```python
from build123d import *

# Parameters (mm, degrees)
BOSS_EXTRUDE1_DEPTH = 3
SKETCH2_W           = 30
SKETCH2_H           = 3
BOSS_EXTRUDE2_DEPTH = 24
SKETCH5_R           = 3.3
CUT_EXTRUDE1_DEPTH  = 10


with BuildPart() as part:
    # Sketch1 → Boss-Extrude1 (new body)
    with BuildSketch(Plane.XZ.offset(-12)):
        Polygon((15, 0), (15, 33), (-15, 3), (-15, 0), align=None)
    extrude(amount=-BOSS_EXTRUDE1_DEPTH)

    # Sketch2 → Boss-Extrude2 (add)
    with BuildSketch(Plane.XZ.offset(-12)):
        with Locations((0, 1.5)):
            Rectangle(SKETCH2_W, SKETCH2_H)
    extrude(amount=BOSS_EXTRUDE2_DEPTH)

    # Sketch5 → Cut-Extrude1 (cut)
    with BuildSketch(Plane(origin=(0, 0, 0), x_dir=(-1, 0, 0), z_dir=(0, 0, -1))):
        with Locations((-9, 3)):
            Circle(SKETCH5_R)
        with Locations((9, 3)):
            Circle(SKETCH5_R)
    extrude(amount=-CUT_EXTRUDE1_DEPTH, mode=Mode.SUBTRACT)


solid = part.part
```
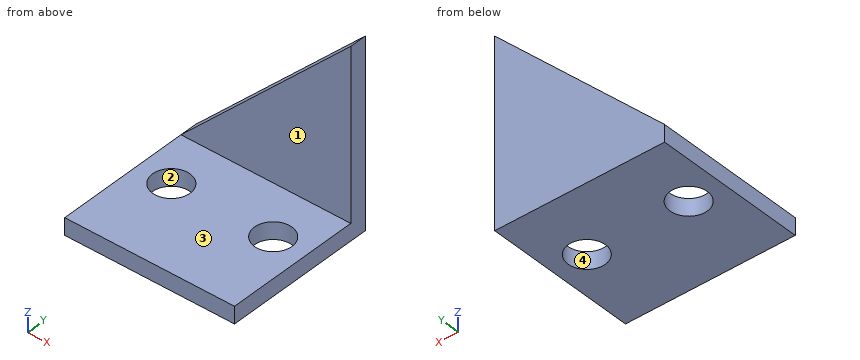
The model under review builds one solid part; all positions refer to its coordinate system, in mm. Face numbers are marked on the shaded views. A direction names the side the tool comes from. Give positions to 0.01 mm unless a question says otherwise; leave off trailing zeros. Write each loop counter-clockwise with the first axis right and the second up, starting at its lowest first coordinate (ties: lowest second). Pieces come first, ordered by that corner, then holes. Notation, with made-up numbers: (46.5, 30.25) - (84.5, 30.25) arc R24 cw to (84.5, 53.25) - close; hole circle Ø5 at (24, 80.5). An arc over 180 degrees is marked (long way). Answer in a Markdown table with one row per item. Add a question column.
1. Draft analysis for pull direction X (two halves, no side actions). For the marked faces 1 and 2, state which applies: +X half, -X half, draft (parallel to the pull), parting line (faces both ways), or undercut.
2. We need section C-C on x = -9. Write out the cut boundary in (y, z).
3. We need section A-A on y = 3. Write out the cut boundary in (x, z), then the cut area to 3 significant figures.
4. Wall thickness on line 1 along Y through (x, z) = (9, 1.15); line 2 along Z through (x, y) = (3, -0.5); line 3 along Y through (x, z) = (4, 21): over which ranges is each line inside the solid? List them lowest first. Write a range as [from, to].
5. We need section B-B on x = 9. Write out the cut boundary in (y, z).
6. Tool access review of the marked faces 3 and 4: name each direction out of +Z, -Z, +X, -X, +Y, -Y from which nothing blocks a thin tool from reaching the whole face with its end or side.
7. We need section D-D on x = -2. Write out the cut boundary in (y, z), then the cut area to 3 significant figures.
8. Insertion check: P1, Ø5, axis at x = -4, z = 16.5, coming from the -Y side; P2, Ø10.5, axis at x = -9, y = 3, coming from the +Z side. Each pin has a flat end and moves straight along its axis. Give the tip position at first contact, or say it passes through.
Ans:
| question | item | result |
|---|---|---|
| 1 | face 1 | draft |
| 1 | face 2 | undercut |
| 2 | outline | (-12, 0) - (-0.3, 0) - (-0.3, 3) - (-12, 3) - close; (6.3, 0) - (15, 0) - (15, 9) - (12, 9) - (12, 3) - (6.3, 3) - close |
| 3 | outline | (-15, 0) - (-12.3, 0) - (-12.3, 3) - (-15, 3) - close; (-5.7, 0) - (5.7, 0) - (5.7, 3) - (-5.7, 3) - close; (12.3, 0) - (15, 0) - (15, 3) - (12.3, 3) - close |
| 3 | area | 50.4 mm^2 |
| 4 | line 1 | y = [-12, -0.3], [6.3, 15] |
| 4 | line 2 | z = [0, 3] |
| 4 | line 3 | y = [12, 15] |
| 5 | outline | (-12, 0) - (-0.3, 0) - (-0.3, 3) - (-12, 3) - close; (6.3, 0) - (15, 0) - (15, 27) - (12, 27) - (12, 3) - (6.3, 3) - close |
| 6 | face 3 | +Z, +X, -X, -Y |
| 6 | face 4 | +Z, -Z |
| 7 | outline | (-12, 0) - (15, 0) - (15, 16) - (12, 16) - (12, 3) - (-12, 3) - close |
| 7 | area | 120 mm^2 |
| 8 | P1 | stops at y = 12 |
| 8 | P2 | stops at z = 3 |
